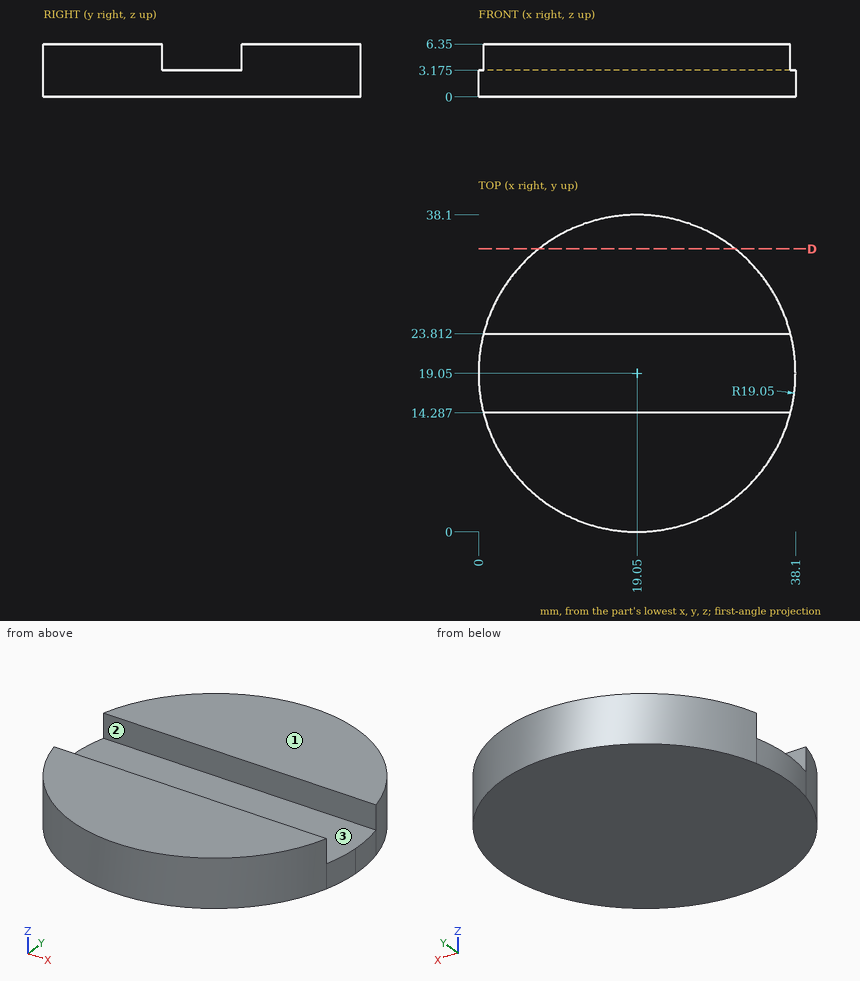
Here's the drawing with two shaded views (mm, measured from the low corner). I have some questions. Coordinates: 2 decimals unless noted, no trailing zeros. Order: outer loops, then holes, each group sorted by start corner. A loop starts at its lowest first (then second) coordinate and runs counter-clockwise, first axis right, second up.
Q1. Please list where these lines run through material, in increasing order: L1, parallel to Z at x = 9.5, y = 21 (1 decimal); L2, parallel to Y at x = 24, z = 3.75 (1 decimal); L3, parallel to X at y = 7, z = 1.5 (1 decimal).
Q2. Suppose I cut it at D-D on y = 34. Please give me the cut outline in (x, z), and give its area (3 significant figures).
Q3. Will these pins go through, and if not, where does the flat tip stop? pin 1 (1.5 mm diameter, centred on x = 7, z = 1.5, fed in from -Y); pin 2 (1 mm diameter, centred on x = 21.5, z = 5, fed in from +Y); pin 3 (3.5 mm diameter, centred on x = 14.5, z = 5, fed in from -Y); pin 4 (8 mm diameter, centred on x = 19, y = 16, fed in from +Z).
Q4. Thinking about a two-plate mould opening in Y: for the marked faces 1, 2 and 3, which applies, released by +Y, released by -Y, zero draft, split by the parting line, or undercut?
Answer:
1. L1: z = 0 to 3.2
1. L2: y = 0.7 to 14.3, 23.8 to 37.4
1. L3: x = 4.3 to 33.8
2. outline: (7.24, 0) - (30.86, 0) - (30.86, 6.35) - (7.24, 6.35) - close
2. area: 150 mm2
3. pin 1: stops at y = 3.71
3. pin 2: stops at y = 38
3. pin 3: stops at y = 0.21
3. pin 4: stops at z = 6.35
4. face 1: zero draft
4. face 2: undercut
4. face 3: undercut
